The figure shows three views and two pictorial views of one solid part (mm, origin at its lowest corner). Answer the questions. A direction names the side the tool comes from. Give positions to 0.01 mm unless a question says otherwise; leave off trailing zeros. Loops run counter-clockwise (first coordinate to the right, second up) from the corner with the lowest first, then second, coordinate; pieces in that order, holes last. Notation, with made-up numbers: M 60,38 L 70,38 A19 cw 70,42 Z; hole C 23,-13.75 d2. An arc over 180 degrees is marked long. Write item = value, one per line. Start each with the question number.
1. For the marked faces 4 and 5, determine the directions among +Z, -Z, +X, -X, +Y, -Y from which every point of the face is accessible in a straight line to the end or side of a thin tool.
2. Consider L1, parallel to X at y = 17, z = 4.65; L2, parallel to Z at x = 48.5, y = 3.5; L3, parallel to Y at x = 53, z = 3.85. Determine where each line is inside the solid, lowest interval first. Write a range as [from, to].
3. Section C-C on x = 15 is taken. Determine the outline of the cut face in (y, z), plus the area to 3 significant figures.
4. Flat-ended cylindrical pins translate along their axes: pin 1 Ø1 at (y, z) = (10.5, 1.5) entering from -X; pin 2 Ø0.6 at (y, z) = (2.5, 4) entering from +X; pin 3 Ø10.5 at (x, y) = (52, 13.5) entering from -Z. Find the tip coordinate at first contact, or state that the pin passes through.
5. Section A-A on x = 39 is taken. Determine the outline of the cut face in (y, z).
6. Section B-B on y = 14.5 is taken. Determine the outline of the cut face in (x, z), plus the area to 3 significant figures.
7. The mould has two halves that part along X. Classify the marked faces 1, 2 and 3: released by +X, released by -X, zero draft, split by the parting line, or undercut.
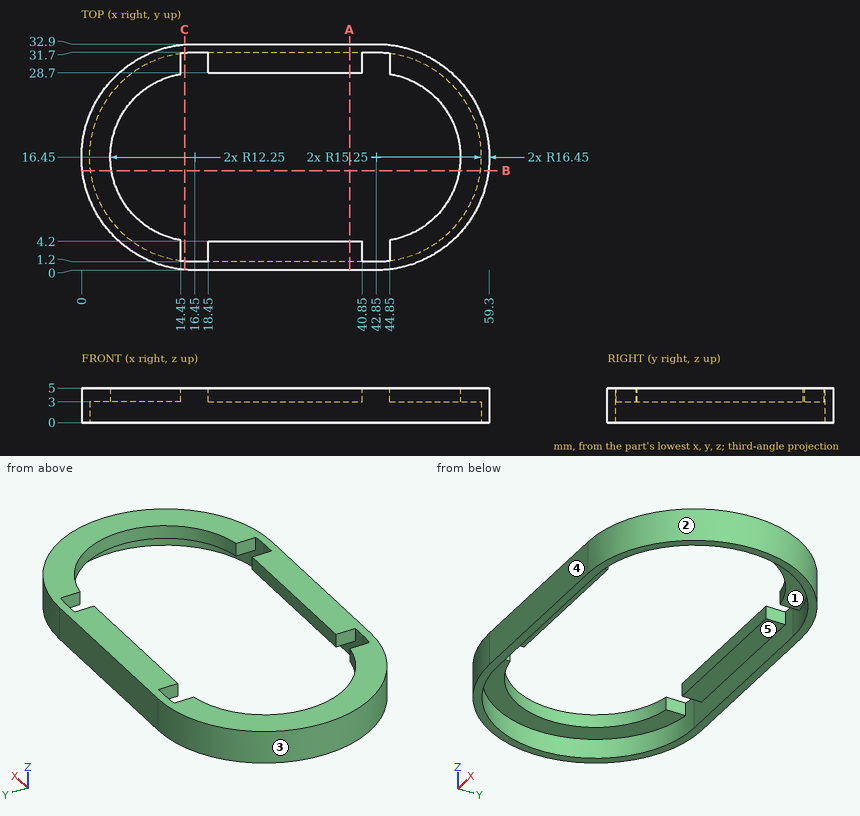
Verdict:
q1.face_4 = +Z, -Z, +X, -X, -Y
q1.face_5 = -Z
q2.L1 = [0.01, 4.21], [55.09, 59.29]
q2.L2 = [3, 5]
q2.L3 = [3.5, 9.59], [23.31, 29.4]
q3.outline = M 0.06,0 L 1.27,0 L 1.27,5 L 0.06,5 Z; M 31.63,0 L 32.84,0 L 32.84,5 L 31.63,5 Z
q3.area = 12.1 mm2
q4.pin_1 = 0.93
q4.pin_2 = 52.03
q4.pin_3 = 3
q5.outline = M 0,0 L 1.2,0 L 1.2,3 L 4.2,3 L 4.2,5 L 0,5 Z; M 28.7,3 L 31.7,3 L 31.7,0 L 32.9,0 L 32.9,5 L 28.7,5 Z
q6.outline = M 0.12,0 L 1.33,0 L 1.33,3 L 4.36,3 L 4.36,5 L 0.12,5 Z; M 54.94,3 L 57.97,3 L 57.97,0 L 59.18,0 L 59.18,5 L 54.94,5 Z
q6.area = 24.2 mm2
q7.face_1 = undercut
q7.face_2 = released by +X
q7.face_3 = released by -X
